Verification items for the finished model (mm, model axes). Coordinates: 2 decimals unless noted, no trailing zeros. Order: outer loops, then holes, each group sorted by start corner. A loop starts at its lowest first (then second) coordinate and runs counter-clockwise, first axis right, second up. Notation, with made-up numbers: (36, 43) -> (83, 43) arc R18 ccw to (83, 61) -> close; hole circle Ø11 at (41.5, -37.5). An arc over 180 degrees is marked (long way). Use CSV: the item, a comma, the result in double quotes. Start each with the question number.
1) Scan lines: line 1 along X through (y, z) = (0, 27); line 2 along X through (y, z) = (-3.25, 117); line 3 along Y through (x, z) = (-4.75, 97). Record each from-to range of solid material in increasing order.
2) Sectioned sample at A-A on z = 177.5. Record the boundary of the cut face in (x, y).
3) Go/stop test with flat-tipped pins: pin 1 (2 mm diameter, centred on y = 2.5, z = 43.5, fed in from -X); pin 2 (4 mm diameter, centred on y = -5.5, z = 140.5, fed in from -X); pin 3 (4 mm diameter, centred on x = 2, z = 166, fed in from -Y). Record where each tip stops, or that it passes through.
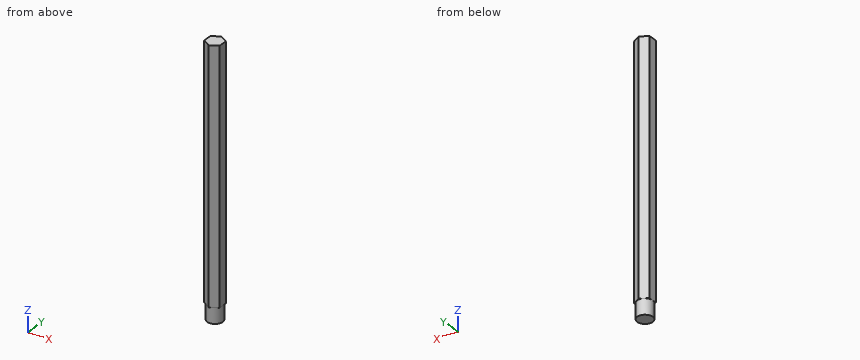
from build123d import *

# Parameters (mm, degrees)
BOSS_EXTRUDE1_DEPTH = 203.2
SKETCH2_R           = 6.35
BOSS_EXTRUDE2_DEPTH = 12.7


with BuildPart() as part:
    # Sketch1 → Boss-Extrude1 (new body)
    with BuildSketch(Plane.XY):
        Polygon((6.217819023, -3.88613689), (6.474402781, 3.441720786), (0.256583757, 7.327857675), (-6.217819023, 3.88613689), (-6.474402781, -3.441720786), (-0.256583757, -7.327857675), align=None)
    extrude(amount=BOSS_EXTRUDE1_DEPTH)

    # Sketch2 → Boss-Extrude2 (add)
    with BuildSketch(Plane(origin=(0, 0, 0), x_dir=(-1, 0, 0), z_dir=(0, 0, -1))):
        Circle(SKETCH2_R)
    extrude(amount=BOSS_EXTRUDE2_DEPTH)


solid = part.part
Answers follow:
1,line 1,"x = -6.35 to 6.35"
1,line 2,"x = -6.47 to 6.24"
1,line 3,"y = -4.52 to 4.67"
2,outline,"(-6.47, -3.44) -> (-0.26, -7.33) -> (6.22, -3.89) -> (6.47, 3.44) -> (0.26, 7.33) -> (-6.22, 3.89) -> close"
3,pin 1,"stops at x = -6.3"
3,pin 2,"stops at x = -6.38"
3,pin 3,"stops at y = -7.19"
